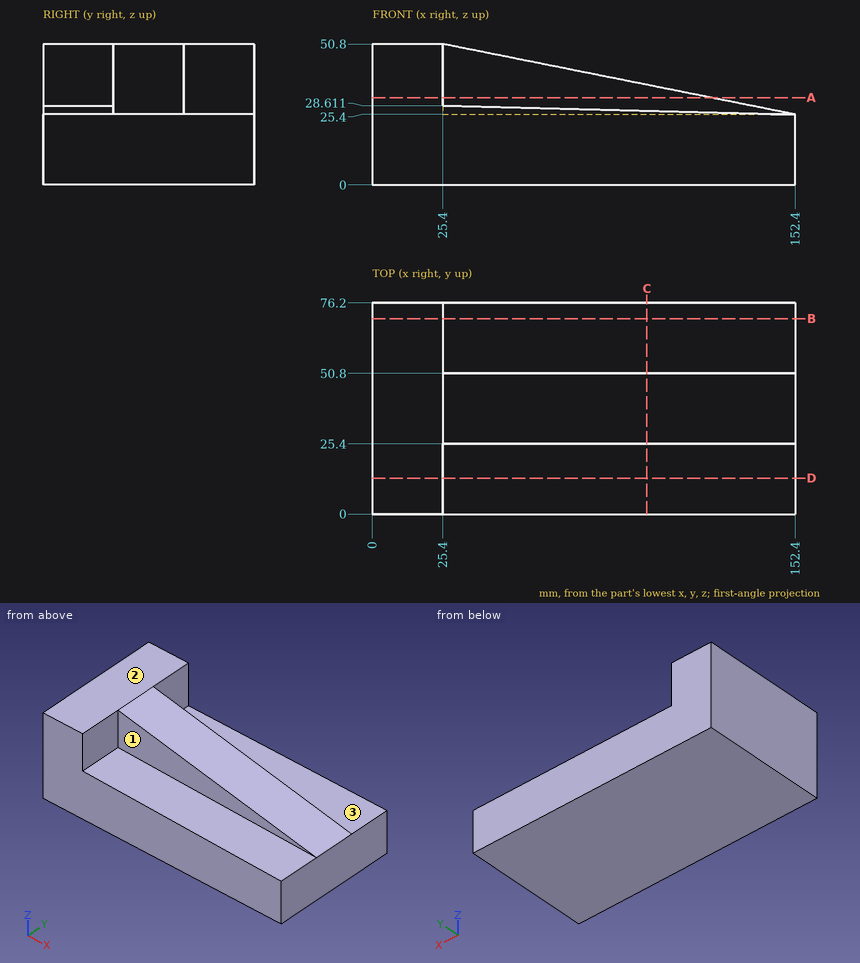
The drawing under review shows one solid part. Ordinate dimensions are in mm from its lowest x, y, z. A direction names the side the tool comes from. Round coordinates to 2 decimals unless told otherwise and drop trailing zeros. Loops run counter-clockwise (first coordinate to the right, second up) from the corner with the lowest first, then second, coordinate; pieces in that order, holes last.
Item 1: For line 1 (Z direction, x = 109.5, y = 55.5); line 2 (Y direction, x = 88, z = 35.5), list the stretches that pass through material, from the lowest coordinate up.
Determined:
line 1: z = 0 to 25.4
line 2: y = 25.4 to 50.8
Item 2: Take a section at C-C (x = 99). Write out the cut boundary in (y, z).
Determined:
outline: (0, 0) - (76.2, 0) - (76.2, 25.4) - (50.8, 25.4) - (50.8, 36.08) - (25.4, 36.08) - (25.4, 26.75) - (0, 26.75) - close
Item 3: Clearance check with flat-ended pins moving along their axes: pin 1 Ø2 at (y, z) = (40, 38.5) entering from -X; pin 2 Ø3 at (y, z) = (62, 33) entering from +X; pin 3 Ø20.5 at (x, y) = (62.5, 63) entering from +Z; pin 4 Ø12.5 at (x, z) = (120.5, 34) entering from +Y. State where each tip first meets the part, or that it passes through.
Determined:
pin 1: stops at x = 0
pin 2: stops at x = 25.4
pin 3: stops at z = 25.4
pin 4: stops at y = 50.8
Item 4: Take a section at A-A (z = 31.5). Write out the cut boundary in (x, y), then the cut area to 3 significant figures.
Determined:
outline: (0, 0) - (25.4, 0) - (25.4, 25.4) - (121.9, 25.4) - (121.9, 50.8) - (25.4, 50.8) - (25.4, 76.2) - (0, 76.2) - close
area: 4,390 mm2
Item 5: Take a section at B-B (y = 70.5). Write out the cut boundary in (x, z).
Determined:
outline: (0, 0) - (152.4, 0) - (152.4, 25.4) - (25.4, 25.4) - (25.4, 50.8) - (0, 50.8) - close
Item 6: For the marked faces 1, 2 and 3, list the 3-axis set-ups (+Z, -Z, +X, -X, +Y, -Y) from which the entire face can be reached by the end or side of a thin tool; tool diameter is ignored.
Determined:
face 1: +Z, +X, -Y
face 2: +Z, +X, -X, +Y, -Y
face 3: +Z, +X, +Y
Item 7: Take a section at D-D (y = 13). Write out the cut boundary in (x, z), then the cut area to 3 significant figures.
Determined:
outline: (0, 0) - (152.4, 0) - (152.4, 25.4) - (25.4, 28.61) - (25.4, 50.8) - (0, 50.8) - close
area: 4,720 mm2
